The model under review builds one solid part; all positions refer to its coordinate system, in mm. Face numbers are marked on the shaded views. A direction names the side the tool comes from. Round coordinates to 2 decimals unless told otherwise and drop trailing zeros. Loops run counter-clockwise (first coordinate to the right, second up) from the corner with the lowest first, then second, coordinate; pieces in that order, holes last. Notation, with made-up numbers: (-13, 24) - (20, 24) arc R25 ccw to (20, 42) - close; hole circle Ø11 at (72.5, -36). An arc over 180 degrees is marked (long way). Answer as CSV lines item,"result".
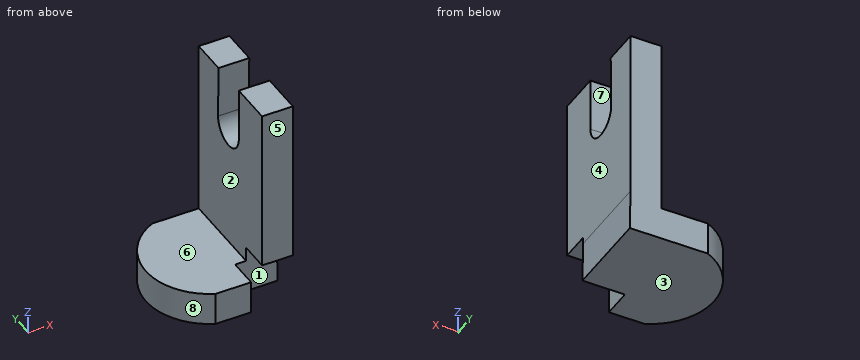
from build123d import *

# Parameters (mm, degrees)
F1_DEPTH      = 15.494
F1_DEPTH_BACK = 13.716
F3_DEPTH      = 25.4
F5_DEPTH      = 25.4
F7_DEPTH      = 7.366


with BuildPart() as f1:
    # F0 (on Front) → F1 (new body, two sides)
    with BuildSketch(Plane.XZ) as f1_sk:
        Polygon((10.631341, -17.505052), (10.44804, -7.240309), (10.44804, 35.468351), (2.74667, 35.468351), (2.74667, -9.236218), (-20.529484, -9.236218), (-20.529484, -17.505052), align=None)
    extrude(amount=F1_DEPTH)
    extrude(f1_sk.sketch, amount=-F1_DEPTH_BACK)

    # F2 (on face) → F3 (cut)
    with BuildSketch(Plane.YZ.offset(10.44804)):
        with BuildLine():
            ThreePointArc((4.782288, 22.142286), (-0.035854, 26.85327), (-4.782825, 22.070579))
            ThreePointArc((-4.782825, 22.070579), (0, 17.287754), (4.782825, 22.070579))
            ThreePointArc((4.782825, 22.070579), (4.782691, 22.106434), (4.782288, 22.142286))
        make_face()
        with BuildLine():
            Line((-4.782825, 35.468351), (-4.782825, 22.070579))
            ThreePointArc((-4.782825, 22.070579), (-0.035854, 26.85327), (4.782288, 22.142286))
            Line((4.782288, 22.142286), (4.582474, 35.468351))
            Line((4.582474, 35.468351), (-4.782825, 35.468351))
        make_face()
    extrude(amount=-F3_DEPTH, mode=Mode.SUBTRACT)

    # F4 (on face) → F5 (cut)
    with BuildSketch(Plane.XY.offset(-9.236218)):
        with BuildLine():
            ThreePointArc((-8.891407, -15.494), (-18.403713, -0.889), (-8.891407, 13.716))
            Line((-8.891407, 13.716), (-20.529484, 13.716))
            Line((-20.529484, 13.716), (-20.529484, -15.494))
            Line((-20.529484, -15.494), (-8.891407, -15.494))
        make_face()
    extrude(amount=-F5_DEPTH, mode=Mode.SUBTRACT)

    # F6 (on face) → F7 (cut)
    with BuildSketch(Plane.XZ.offset(15.494)):
        Polygon((10.44804, -5.590619), (2.74667, -5.590619), (2.74667, -9.236218), (0, -9.236218), (0, -17.505052), (10.631341, -17.505052), (10.44804, -7.240309), align=None)
    extrude(amount=-F7_DEPTH, mode=Mode.SUBTRACT)


solid = f1.part
1. Take a section at A-A (x = 8.5). State the section outline as (y, z) points.
Numbers:
outline,"(-15.49, -5.59) - (-8.13, -5.59) - (-8.13, -17.51) - (13.72, -17.51) - (13.72, 35.47) - (4.58, 35.47) - (4.78, 22.14) arc R4.78 cw to (4.78, 22.07) arc R4.78 cw to (-4.78, 22.07) - (-4.78, 35.47) - (-15.49, 35.47) - close"
2. Take a section at C-C (y = -9.5). State the section outline as (x, z) points, plus the area to 3 significant figures.
Numbers:
outline,"(-15.88, -17.51) - (0, -17.51) - (0, -9.24) - (-15.88, -9.24) - close; (2.75, -5.59) - (10.45, -5.59) - (10.45, 35.47) - (2.75, 35.47) - close"
area,"448 mm²"
3. Wall thickness on probe 1 along Z at (x, y) = (2.5, 4.75); probe 2 along X at (y, z) = (1, 0.5); probe 3 along Y at (x, z) = (4.75, 27.5): over which ranges is each line inside the solid? List them lowest first.
Numbers:
probe 1,"z = -17.51 to -9.24"
probe 2,"x = 2.75 to 10.45"
probe 3,"y = -15.49 to -4.78, 4.7 to 13.72"
4. Take a section at B-B (z = 19.5). State the section outline as (x, y) points.
Numbers:
outline,"(2.75, -15.49) - (10.45, -15.49) - (10.45, -4.03) - (2.75, -4.03) - close; (2.75, 4.03) - (10.45, 4.03) - (10.45, 13.72) - (2.75, 13.72) - close"
5. Take a section at D-D (y = 0). State the section outline as (x, z) points, plus the area to 3 significant figures.
Numbers:
outline,"(-18.38, -17.51) - (10.63, -17.51) - (10.45, -7.24) - (10.45, 17.29) - (2.75, 17.29) - (2.75, -9.24) - (-18.38, -9.24) - close"
area,"444 mm²"
6. Draft analysis for pull direction Y (two halves, no side actions). For the marked faces 6, 7 and 8, state which applies: +Y half, -Y half, draft (parallel to the pull), parting line (faces both ways), or undercut.
Numbers:
face 6,"draft"
face 7,"undercut"
face 8,"parting line"
7. Tool access review of the marked faces 1, 2, 3, 4 and 5: name each direction out of +Z, -Z, +X, -X, +Y, -Y from which nothing blocks a thin tool from reaching the whole face with its end or side.
Numbers:
face 1,"-Z, +X, -Y"
face 2,"+Z, -X, +Y, -Y"
face 3,"-Z, +X, -X, +Y, -Y"
face 4,"+Z, +X, +Y, -Y"
face 5,"+Z, -Z, +X, -X, -Y"
8. Clearance check with flat-ended pins moving along their axes: pin 1 (4 mm diameter, centred on x = -15, y = -8.5, fed in from +Z); pin 2 (12 mm diameter, centred on y = 2, z = 15.5, fed in from -X); pin 3 (6 mm diameter, centred on y = -12.5, z = -12.5, fed in from +X). State where each tip first meets the part, or that it passes through.
Numbers:
pin 1,"stops at z = -9.24"
pin 2,"stops at x = 2.75"
pin 3,"stops at x = 0"
